Read the model definition and answer for the solid it produces. Units are mm, in the model's axes. Face numbers are marked on the shaded views. A direction names the side the tool comes from. Coordinates: 2 decimals unless noted, no trailing zeros. Loops run counter-clockwise (first coordinate to the right, second up) from the corner with the lowest first, then second, coordinate; pieces in that order, holes last.
from build123d import *

# Parameters (mm, degrees)
F0_W     = 73.782653
F0_H     = 66.537239
F1_DEPTH = 56.762496
F2_R     = 25.49506
F3_T     = -2.54


with BuildPart() as f1:
    # F0 (on Top) → F1 (new body)
    with BuildSketch(Plane.XY):
        with Locations((-2.154655, 33.268619)):
            Rectangle(F0_W, F0_H)
    extrude(amount=F1_DEPTH)

    # F2
    f2_edges = [f1.edges().sort_by_distance(p)[0] for p in [
        (-2.154656, 66.537239, 56.762496),
        (34.736671, 66.537239, 28.381248),
        (34.736671, 33.268619, 56.762496),
    ]]
    fillet(f2_edges, radius=F2_R)

    # F3
    f3_openings = [f1.faces().sort_by_distance(p)[0] for p in [
        (-3.066985, 32.462235, 0),
    ]]
    offset(amount=F3_T, openings=f3_openings)


solid = f1.part
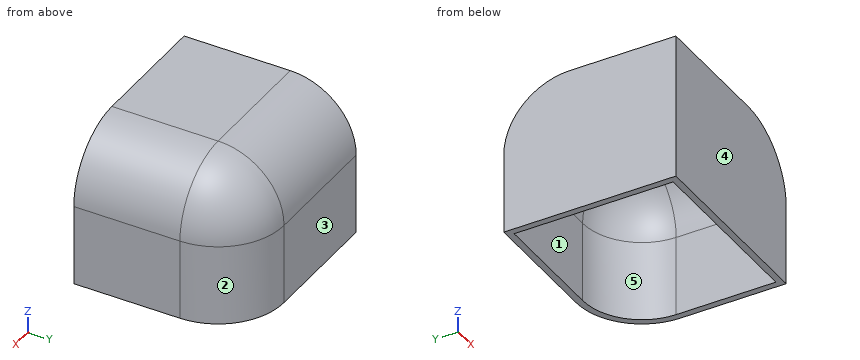
Q1. A cutting plane is placed at B-B (y = 7). Give the vertices of the cut face in (x, z).
Findings below:
outline: (-39.05, 0) - (-36.51, 0) - (-36.51, 54.22) - (9.24, 54.22) arc R22.96 cw to (32.2, 31.27) - (32.2, 0) - (34.74, 0) - (34.74, 31.27) arc R25.5 ccw to (9.24, 56.76) - (-39.05, 56.76) - close
Q2. Flat-ended cylindrical pins translate along their axes: pin 1 Ø1.5 at (y, z) = (59.5, 13) entering from +X; pin 2 Ø1 at (x, y) = (21.5, 48.5) entering from +Z; pin 3 Ø19.5 at (x, y) = (-21, 24.5) entering from -Z. Find the tip coordinate at first contact, or state that the pin passes through.
Findings below:
pin 1: stops at x = 27.58
pin 2: stops at z = 52.67
pin 3: stops at z = 54.22
Q3. Determine the mould class of the marked faces 3, 4 and 5 for opening direction Y: +Y half, -Y half, draft (parallel to the pull), parting line (faces both ways), or undercut.
Findings below:
face 3: +Y half
face 4: -Y half
face 5: undercut
Q4. A cutting plane is placed at A-A (z = 11). Give the vertices of the cut face in (x, y).
Findings below:
outline: (-39.05, 0) - (34.74, 0) - (34.74, 41.04) arc R25.5 ccw to (9.24, 66.54) - (-39.05, 66.54) - close; hole (-36.51, 2.54) - (32.2, 2.54) - (32.2, 41.04) arc R22.96 ccw to (9.24, 64) - (-36.51, 64) - close
Q5. A cutting plane is placed at D-D (z = 35.5). Give the vertices of the cut face in (x, y), then the cut area to 3 significant figures.
Findings below:
outline: (-39.05, 0) - (34.38, 0) - (34.38, 41.04) arc R25.14 ccw to (9.24, 66.18) - (-39.05, 66.18) - close; hole (-36.51, 2.54) - (31.8, 2.54) - (31.8, 41.04) arc R22.56 ccw to (9.24, 63.6) - (-36.51, 63.6) - close
area: 662 mm2
Q6. Straight lines are drawn through the part: probe 1 along X at (y, z) = (6.5, 13); probe 2 along Y at (x, z) = (-16, 27); probe 3 along X at (y, z) = (55.5, 37). For each, find the intervals that lie inside material, in ascending order.
Findings below:
probe 1: x = -39.05 to -36.51, 32.2 to 34.74
probe 2: y = 0 to 2.54, 64 to 66.54
probe 3: x = -39.05 to -36.51, 26.12 to 29.44
Q7. A cutting plane is placed at C-C (x = 1). Give the vertices of the cut face in (y, z).
Findings below:
outline: (0, 0) - (2.54, 0) - (2.54, 54.22) - (41.04, 54.22) arc R22.96 cw to (64, 31.27) - (64, 0) - (66.54, 0) - (66.54, 31.27) arc R25.5 ccw to (41.04, 56.76) - (0, 56.76) - close
Q8. Which of the six approach directions +Z, -Z, +X, -X, +Y, -Y give full straight-line access (tool end or side, diameter ignored) to the marked faces 1 and 2?
Findings below:
face 1: -Z
face 2: +Z, -Z, +X, +Y
